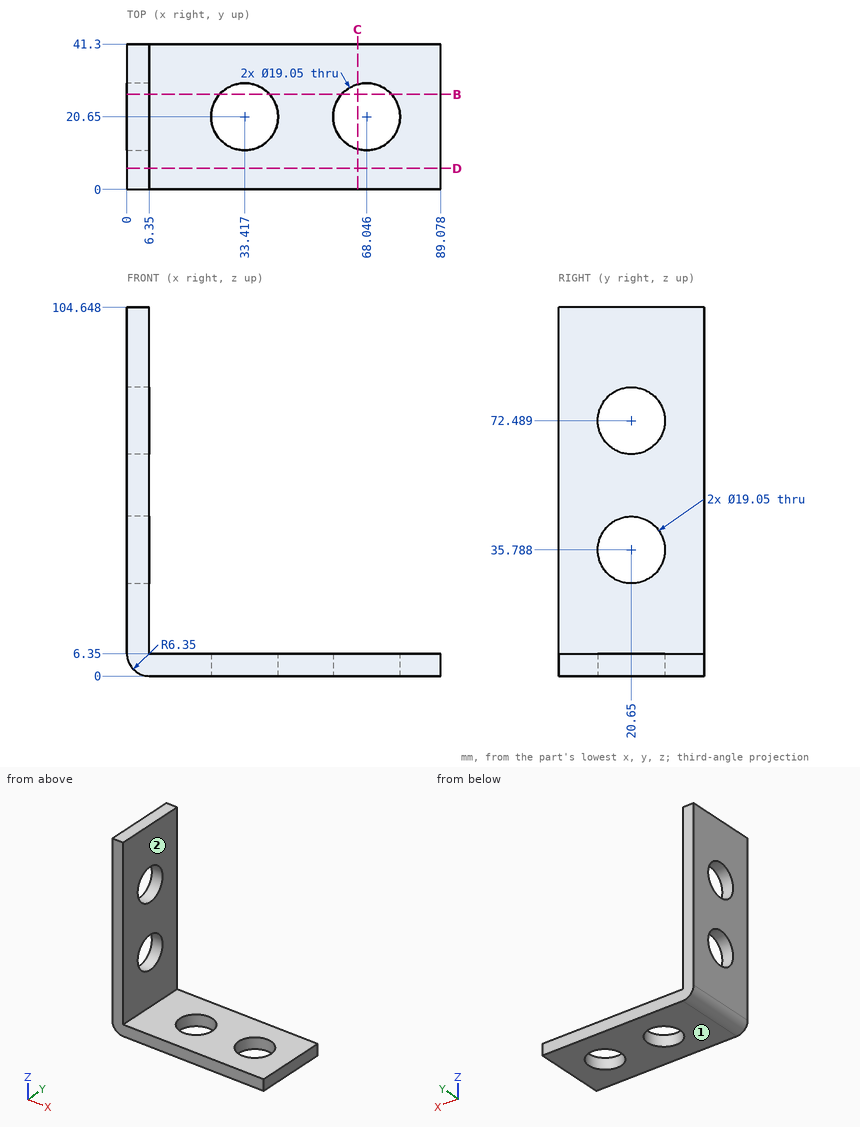
Geometry: see drawing. Coordinates: mm, zero at the bounding-box minimum. A direction names the side the tool comes from. Round coordinates to 2 decimals unless told otherwise and drop trailing zeros. Loops run counter-clockwise (first coordinate to the right, second up) from the corner with the lowest first, then second, coordinate; pieces in that order, holes last. Notation, with made-up numbers: M -8,26.5 L 42,26.5 A31 ccw 42,64.5 Z; hole C -39.5,35 d5. An arc over 180 degrees is marked long. Use a Markdown table: item, result. Add a question column.
1. Contact query for flat-ended pins moving along their axis: pin 1 (20.5 mm diameter, centred on y = 19.5, z = 47.5, fed in from +X); pin 2 (10 mm diameter, centred on x = 27, y = 4.5, fed in from +Z); pin 3 (17 mm diameter, centred on y = 20.65, z = 72.49, fed in from -X); pin 4 (12 mm diameter, centred on y = 19, z = 90, fed in from -X). Output: stop coordinate, or through.
2. Ray query, line 1 along Z through (x, y) = (51, 20.5). Return the intervals inside material, ascending. Write a range as [from, to].
3. Cut plane C-C, the plane x = 65.5. Output: boundary loops of the cut face in (y, z), and give its area (3 significant figures).
4. Set-up query: the marked faces 1 and 2. Return all of +Z, -Z, +X, -X, +Y, -Y with unobstructed straight access to the full face (end or side cutting, diameter ignored); none if empty.
5. Cut plane D-D, the plane y = 6. Output: boundary loops of the cut face in (x, z).
6. Cut plane B-B, the plane y = 27. State how many separate pieces and enclosed holes the cut face has.
Solution:
| question | item | result |
|---|---|---|
| 1 | pin 1 | stops at x = 6.35 |
| 1 | pin 2 | stops at z = 6.35 |
| 1 | pin 3 | passes through |
| 1 | pin 4 | stops at x = 0 |
| 2 | line 1 | z = [0, 6.35] |
| 3 | outline | M 0,0 L 11.47,0 L 11.47,6.35 L 0,6.35 Z; M 29.83,0 L 41.3,0 L 41.3,6.35 L 29.83,6.35 Z |
| 3 | area | 146 mm2 |
| 4 | face 1 | -Z, +X, -X, +Y, -Y |
| 4 | face 2 | +Z, +X, +Y, -Y |
| 5 | outline | M 0,6.35 A6.35 ccw 6.35,0 L 89.08,0 L 89.08,6.35 L 6.35,6.35 L 6.35,104.65 L 0,104.65 Z |
| 6 | separate pieces | 5 |
| 6 | enclosed holes | 0 |
